Source: CAD feature listing. Evaluate the final solid. Frame: model axes, mm. Give positions to 0.01 mm unless a question says otherwise; leave off trailing zeros. Order: outer loops, then holes, each group sorted by start corner. A loop starts at its lowest first (then second) coordinate and runs counter-clockwise, first axis right, second up. Notation, with made-up numbers: (31.5, 48.25) -> (69.5, 48.25) arc R23 ccw to (69.5, 77.25) -> close; hole circle Ø1 at (58.5, 45.25). An arc over 180 degrees is marked (long way). Answer in a Markdown table with one row per item.
```python
from build123d import *

# Parameters (mm, degrees)
BOSS_EXTRUDE1_DEPTH         = 12.7
F_1_4_20_TAPPED_HOLE1_D     = 5.1054
F_1_4_20_TAPPED_HOLE1_DEPTH = 19.05
F_1_4_20_TAPPED_HOLE1_TIP   = 1.533816902


with BuildPart() as part:
    # Sketch1 → Boss-Extrude1 (new body)
    with BuildSketch(Plane(origin=(0, 0, 0), x_dir=(1, 0, 0), z_dir=(0, 1, 0))):
        with BuildLine():
            Line((-12.7, 121.25), (-12.7, 0))
            ThreePointArc((-12.7, 0), (-4.670226784, -11.810122005), (9.265193981, -8.685976081))
            Line((9.265193981, -8.685976081), (122.935193981, 112.564023919))
            ThreePointArc((122.935193981, 112.564023919), (125.323366386, 126.298668328), (113.67, 133.95))
            Line((113.67, 133.95), (0, 133.95))
            ThreePointArc((0, 133.95), (-8.980256121, 130.230256121), (-12.7, 121.25))
        make_face()
    extrude(amount=BOSS_EXTRUDE1_DEPTH)

    # 1/4-20 Tapped Hole1
    with Locations(Plane(origin=(10.018427162, 12.7, -35.98129538), x_dir=(0, 0, 1), z_dir=(0, 1, 0))):
        with Locations((0, 0), (-72.954283318, 68.393512452)):
            Hole(F_1_4_20_TAPPED_HOLE1_D / 2, depth=F_1_4_20_TAPPED_HOLE1_DEPTH)
            with Locations((0, 0, -(F_1_4_20_TAPPED_HOLE1_DEPTH + F_1_4_20_TAPPED_HOLE1_TIP / 2))):  # 118° drill point
                Cone(0, F_1_4_20_TAPPED_HOLE1_D / 2, F_1_4_20_TAPPED_HOLE1_TIP, mode=Mode.SUBTRACT)


solid = part.part
```
(1) Section query A-A (y = 3.5). Return the cut outline in (x, z), plus the area to 3 significant figures.
A:
| item | result |
|---|---|
| outline | (-12.7, -121.25) arc R12.7 ccw to (0, -133.95) -> (113.67, -133.95) arc R12.7 ccw to (122.94, -112.56) -> (9.27, 8.69) arc R12.7 ccw to (-12.7, 0) -> close; hole circle Ø5.11 at (10.02, -35.98); hole circle Ø5.11 at (78.41, -108.94) |
| area | 12,500 mm^2 |
(2) Section query C-C (z = -66.5). Return the cut outline in (x, y), plus the area to 3 significant figures.
A:
| item | result |
|---|---|
| outline | (-12.7, 0) -> (79.75, 0) -> (79.75, 12.7) -> (-12.7, 12.7) -> close |
| area | 1,170 mm^2 |
(3) Pull-direction query (X, two-part tool) for faces 1 (the cylindrical face through (-4.87, 6.26, 11.73)), 2 (the cylindrical face through (8.465, 6.261, -33.956)), 3 (the flat face through (40, 12.7, -78)), 4 (the flat face through (65.305, 6.261, -51.09)); classes: +X half, -X half, draft (parallel to the pull), parting line (faces both ways), or undercut.
A:
| item | result |
|---|---|
| face 1 | parting line |
| face 2 | undercut |
| face 3 | draft |
| face 4 | +X half |
(4) First-contact query: pin 1 Ø5 at (x, y) = (30, 11) entering from +Z; pin 2 Ø2 at (y, z) = (6.5, -11) entering from +X; pin 3 Ø3 at (y, z) = (2, -100) entering from +X. Flat tips, straight axial feed; report the tip coordinate or a pass-through.
A:
| item | result |
|---|---|
| pin 1 | stops at z = -10.76 |
| pin 2 | stops at x = 28.66 |
| pin 3 | stops at x = 112.56 |
(5) Ray query, probe 1 along Z at (x, y) = (-0.5, 10.75); probe 2 along Z at (x, y) = (10, 2); probe 3 along X at (y, z) = (4, 5). Return the intervals inside material, ascending.
A:
| item | result |
|---|---|
| probe 1 | z = -133.94 to 12.69 |
| probe 2 | z = -133.95 to -38.53, -33.43 to 7.9 |
| probe 3 | x = -11.67 to 12.72 |
(6) Section query B-B (x = 44.5). Return the cut outline in (y, z).
A:
| item | result |
|---|---|
| outline | (0, -133.95) -> (12.7, -133.95) -> (12.7, -28.9) -> (0, -28.9) -> close |
